from build123d import *

# Parameters (mm, degrees)
SKETCH1_W          = 12
SKETCH1_H          = 12
EXTRUDE1_DEPTH     = 7.5
SKETCH2_R          = 2.5
CUT_EXTRUDE1_DEPTH = 13
SKETCH3_R          = 2.5
CUT_EXTRUDE2_DEPTH = 13
FILLET1_R          = 4


with BuildPart() as part:
    # Sketch1 → Extrude1 (new body, symmetric)
    with BuildSketch(Plane.XY):
        Rectangle(SKETCH1_W, SKETCH1_H)
    extrude(amount=EXTRUDE1_DEPTH, both=True)

    # Sketch2 → Cut-Extrude1 (cut, through all)
    with BuildSketch(Plane(origin=(0, 6, 0), x_dir=(1, 0, 0), z_dir=(0, 1, 0))):
        with Locations((0, 4)):
            Circle(SKETCH2_R)
    extrude(amount=-CUT_EXTRUDE1_DEPTH, mode=Mode.SUBTRACT)

    # Sketch3 → Cut-Extrude2 (cut, through all)
    with BuildSketch(Plane(origin=(6, 0, 0), x_dir=(0, 0, -1), z_dir=(1, 0, 0))):
        with Locations((-4, 0)):
            Circle(SKETCH3_R)
    extrude(amount=-CUT_EXTRUDE2_DEPTH, mode=Mode.SUBTRACT)

    # Fillet1
    fillet1_edges = [part.edges().sort_by_distance(p)[0] for p in [
        (0, 6, 7.5),
        (6, 0, -7.5),
        (-6, 0, -7.5),
        (0, -6, 7.5),
    ]]
    fillet(fillet1_edges, radius=FILLET1_R)


solid = part.part
Input: part model. Units: mm. Frame: model coordinates. Coordinates: 2 decimals unless noted, no trailing zeros. Order: outer loops, then holes, each group sorted by start corner. A loop starts at its lowest first (then second) coordinate and runs counter-clockwise, first axis right, second up. Notation, with made-up numbers: M 76.25,-5.75 L 128.25,-5.75 A18 ccw 128.25,11.25 Z; hole C 23.5,87 d7. An arc over 180 degrees is marked long. Write item = value, one per line. Start each with the question number.
(1) Section A-A on x = 0. Output: boundary loops of the cut face in (y, z), and give its area (3 significant figures).
(2) Pull-direction query (Y, two-part tool) for faces 1 (the flat face through (0, -6, -1)), 2 (the cylindrical face through (0.084, 0.751, 1.615)), 3 (the flat face through (0, 6, -1)), 4 (the flat face through (0, 0, 7.5)); classes: released by +Y, released by -Y, zero draft, split by the parting line, or undercut.
(3) Section B-B on z = 5.25. Output: boundary loops of the cut face in (x, y).
(4) Section D-D on y = 4.75. Output: boundary loops of the cut face in (x, z).
(5) Line query: line 1 along Z through (x, y) = (0, -1); line 2 along Z through (x, y) = (-2, 1.25); line 3 along X through (y, z) = (2.75, -4). Output: solid intervals per line, ascending. Write a range as [from, to].
(6) Section C-C on y = 0.75. Output: boundary loops of the cut face in (x, z).
Result set:
q1.outline = M -6,-7.5 L 6,-7.5 L 6,-6.5 L -6,-6.5 Z; M -6,-1.5 L 6,-1.5 L 6,3.5 A4 ccw 2,7.5 L -2,7.5 A4 ccw -6,3.5 Z; hole C 0,4 d5
q1.area = 93.5 mm²
q2.face_1 = released by -Y
q2.face_2 = undercut
q2.face_3 = released by +Y
q2.face_4 = zero draft
q3.outline = M -6,-5.6 L 6,-5.6 L 6,-2.17 L -6,-2.17 Z; M -6,2.17 L 6,2.17 L 6,5.6 L -6,5.6 Z
q4.outline = M -6,-3.5 A4 ccw -2,-7.5 L 2,-7.5 A4 ccw 6,-3.5 L 6,6.4 L -6,6.4 Z; hole C 0,-4 d5
q5.line_1 = [-7.5, -6.5], [-1.5, 1.71], [6.29, 7.5]
q5.line_2 = [-7.5, -5.5], [-2.5, 1.83], [6.17, 7.5]
q5.line_3 = [-5.97, -2.5], [2.5, 5.97]
q6.outline = M -6,-3.5 A4 ccw -2,-7.5 L 2,-7.5 A4 ccw 6,-3.5 L 6,1.62 L -6,1.62 Z; M -6,6.38 L 6,6.38 L 6,7.5 L -6,7.5 Z; hole C 0,-4 d5
